```python
from build123d import *

# Parameters (mm, degrees)
SKETCH_1_W      = 20
SKETCH_1_H      = 41
EXTRUDE_1_DEPTH = 37
SKETCH_2_W      = 2.45
SKETCH_2_H      = 19
EXTRUDE_2_DEPTH = 7
SKETCH_3_W      = 2.45
SKETCH_3_H      = 19
EXTRUDE_3_DEPTH = 7
SKETCH_4_R      = 3
EXTRUDE_4_DEPTH = 7.7
SKETCH_5_R      = 9
EXTRUDE_5_DEPTH = 1.4
SKETCH_7_R      = 6.5
EXTRUDE_6_DEPTH = 0.8


with BuildPart() as part:
    # 草圖1 → 填料-伸長1 (new body)
    with BuildSketch(Plane(origin=(0, 0, 0), x_dir=(0, 0, -1), z_dir=(1, 0, 0))):
        with Locations((-1.083039195, -2.285391089)):
            Rectangle(SKETCH_1_W, SKETCH_1_H)
    extrude(amount=EXTRUDE_1_DEPTH)

    # 草圖2 → 填料-伸長2 (add)
    with BuildSketch(Plane(origin=(0, 18.214608911, 0), x_dir=(1, 0, 0), z_dir=(0, 1, 0))):
        with Locations((30.225, -1.083039195)):
            Rectangle(SKETCH_2_W, SKETCH_2_H)
    extrude(amount=EXTRUDE_2_DEPTH)

    # 草圖3 → 填料-伸長3 (add)
    with BuildSketch(Plane.XZ.offset(22.785391089)):
        with Locations((30.225, 1.083039195)):
            Rectangle(SKETCH_3_W, SKETCH_3_H)
    extrude(amount=EXTRUDE_3_DEPTH)

    # 草圖4 → 填料-伸長4 (add)
    with BuildSketch(Plane(origin=(37, 0, 0), x_dir=(0, 0, -1), z_dir=(1, 0, 0))):
        with Locations(Location((-1.083039195, 9.214608911, 0), (0, 0, 180))):
            Circle(SKETCH_4_R)
    extrude(amount=EXTRUDE_4_DEPTH)

    # 草圖5 → 填料-伸長5 (add)
    with BuildSketch(Plane(origin=(37, 0, 0), x_dir=(0, 0, -1), z_dir=(1, 0, 0))):
        with Locations(Location((-1.083039195, 9.214608911, 0), (0, 0, 90))):
            Circle(SKETCH_5_R)
    extrude(amount=EXTRUDE_5_DEPTH)

    # 草圖7 → 填料-伸長6 (add)
    with BuildSketch(Plane(origin=(38.4, 0, 0), x_dir=(0, 0, -1), z_dir=(1, 0, 0))):
        with Locations((-1.083039195, 9.214608911)):
            Circle(SKETCH_7_R)
    extrude(amount=EXTRUDE_6_DEPTH)


solid = part.part
```
Source: CAD feature listing. Evaluate the final solid. Frame: model axes, mm. A direction names the side the tool comes from. Round coordinates to 2 decimals unless told otherwise and drop trailing zeros. Loops run counter-clockwise (first coordinate to the right, second up) from the corner with the lowest first, then second, coordinate; pieces in that order, holes last. Notation, with made-up numbers: M 45,71.5 L 52,71.5 A7 cw 52,80.5 Z; hole C 59.5,59.25 d8. An arc over 180 degrees is marked long. Use a Markdown table: item, result. Add a question column.
1. Section query B-B on z = 6.5. Return the cut outline in (x, y).
2. Section query D-D on y = -17. Return the cut outline in (x, z), then the cut area to 3 significant figures.
3. Contact query for flat-ended pins moving along their axis: P1, Ø1, axis at x = 34, z = -6.5, coming from the +Y side; P2, Ø12, axis at x = 9.5, z = 3.5, coming from the -Y side; P3, Ø12, axis at y = 4.5, z = -5.5, coming from the +X side; P4, Ø0.7, axis at x = 30.5, y = 22, coming from the -Z side. Output: stop coordinate, or through.
4. Reachability of faces 1 (the flat face through (30, -26, -8.417)), 2 (the flat face through (30, 22, -8.417)), 3 (the flat face through (29, 22, 1)), 4 (the flat face through (29, -26, 1)) from +Z, -Z, +X, -X, +Y, -Y: full face, straight path, thin tool, end or side. Return the list, or none.
5. Line query: line 1 (X direction, y = 11.5, z = -3.75); line 2 (Y direction, x = 25.5, z = 4); line 3 (X direction, y = -11, z = 4.25). Output: solid intervals per line, ascending.
6. Section query C-C on x = 35.5. Return the cut outline in (y, z), then the cut area to 3 significant figures.
7. Section query A-A on y = 1.5. Return the cut outline in (x, z), then the cut area to 3 significant figures.
Reported:
| question | item | result |
|---|---|---|
| 1 | outline | M 0,-22.79 L 29,-22.79 L 29,-29.79 L 31.45,-29.79 L 31.45,-22.79 L 37,-22.79 L 37,2.03 L 38.4,2.03 L 38.4,5.62 L 39.2,5.62 L 39.2,12.81 L 38.4,12.81 L 38.4,16.4 L 37,16.4 L 37,18.21 L 31.45,18.21 L 31.45,25.21 L 29,25.21 L 29,18.21 L 0,18.21 Z |
| 2 | outline | M 0,-8.92 L 37,-8.92 L 37,11.08 L 0,11.08 Z |
| 2 | area | 740 mm² |
| 3 | P1 | stops at y = 18.21 |
| 3 | P2 | stops at y = -22.79 |
| 3 | P3 | stops at x = 44.7 |
| 3 | P4 | stops at z = -8.42 |
| 4 | face 1 | -Z, +X, -X, -Y |
| 4 | face 2 | -Z, +X, -X, +Y |
| 4 | face 3 | +Z, -Z, -X, +Y |
| 4 | face 4 | +Z, -Z, -X, -Y |
| 5 | line 1 | x = 0 to 39.2 |
| 5 | line 2 | y = -22.79 to 18.21 |
| 5 | line 3 | x = 0 to 37 |
| 6 | outline | M -22.79,-8.92 L 18.21,-8.92 L 18.21,11.08 L -22.79,11.08 Z |
| 6 | area | 820 mm² |
| 7 | outline | M 0,-8.92 L 37,-8.92 L 37,-3.55 L 38.4,-3.55 L 38.4,5.72 L 37,5.72 L 37,11.08 L 0,11.08 Z |
| 7 | area | 753 mm² |
